```python
from build123d import *

# Parameters (mm, degrees)
F2_DEPTH = 12.7
F3_R     = 9.525
F4_DEPTH = 12.7
F5_W     = 60
F5_H     = 12.7
F5_W_2   = 12.7
F5_H_2   = 60
F6_DEPTH = 19.05
F7_W     = 203.2
F7_H     = 203.2
F7_W_2   = 184.15
F7_H_2   = 184.15
F8_DEPTH = 152.4


with BuildPart() as f2:
    # F1 (on offset) → F2 (new body)
    with BuildSketch(Plane.XY.offset(304.8)):
        Polygon((50.8, 17.960512), (68.760512, 0), (477.339488, 0), (495.3, 17.960512), (495.3, 337.639488), (477.339488, 355.6), (68.760512, 355.6), (50.8, 337.639488), align=None)
    extrude(amount=-F2_DEPTH)

    # F3 (on face) → F4 (cut)
    with BuildSketch(Plane.XY.offset(304.8)):
        with Locations((396.217286, 302.437495)):
            Circle(F3_R)
        with Locations((396.217286, 42.437495)):
            Circle(F3_R)
        with Locations((136.217286, 302.437495)):
            Circle(F3_R)
        with Locations((136.217286, 42.437495)):
            Circle(F3_R)
    extrude(amount=-F4_DEPTH, mode=Mode.SUBTRACT)

    # F5 (on face) → F6 (join)
    with BuildSketch(Plane.XY.offset(304.8)):
        with Locations((273.05, 331.7875)):
            Rectangle(F5_W, F5_H)
        with Locations((432.4, 172.4375)):
            Rectangle(F5_W_2, F5_H_2)
    extrude(amount=F6_DEPTH)

    # F7 (on face) → F8 (join)
    with BuildSketch(Plane(origin=(0, 0, 292.1), x_dir=(1, 0, 0), z_dir=(0, 0, -1))):
        with Locations((273.05, -177.8)):
            Rectangle(F7_W, F7_H)
        with Locations((273.05, -177.8)):
            Rectangle(F7_W_2, F7_H_2, mode=Mode.SUBTRACT)
    extrude(amount=F8_DEPTH)


solid = f2.part
```
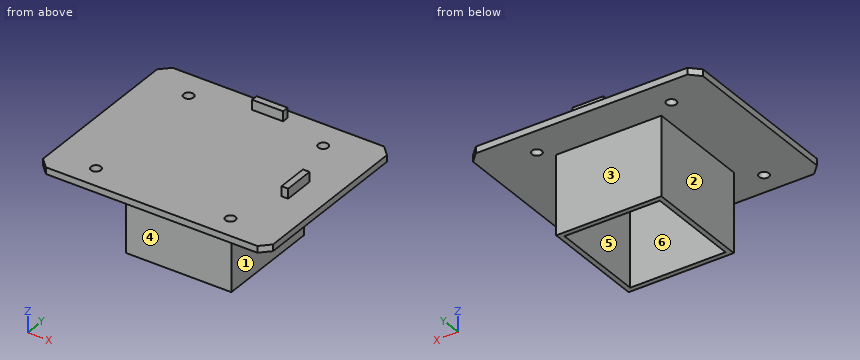
Design review of the part built by this model. Coordinates are the model's own, in mm. Face numbers are marked on the shaded views. A direction names the side the tool comes from. Round coordinates to 2 decimals unless told otherwise and drop trailing zeros. Write each loop counter-clockwise with the first axis right and the second up, starting at its lowest first coordinate (ties: lowest second). Pieces come first, ordered by that corner, then holes. Notation, with made-up numbers: (-27.75, 61) -> (0.25, 61) arc R15 cw to (0.25, 88) -> close; hole circle Ø8 at (84.5, 58.5). An arc over 180 degrees is marked (long way). Answer in a Markdown table with one row per item.
Q1. Take a section at C-C, the plane z = 177.5. State the section outline as (x, y) points (3 decimals).
The answers:
| item | result |
|---|---|
| outline | (171.45, 76.2) -> (374.65, 76.2) -> (374.65, 279.4) -> (171.45, 279.4) -> close; hole (180.975, 85.725) -> (365.125, 85.725) -> (365.125, 269.875) -> (180.975, 269.875) -> close |
Q2. Clearance check with flat-ended pins moving along their axes: pin 1 Ø10 at (y, z) = (79.5, 285.5) entering from -X; pin 2 Ø2 at (x, y) = (116, 230.5) entering from -Z; pin 3 Ø8 at (x, y) = (195.5, 119.5) entering from +Z. State where each tip first meets the part, or that it passes through.
The answers:
| item | result |
|---|---|
| pin 1 | x = 171.45 |
| pin 2 | z = 292.1 |
| pin 3 | z = 304.8 |
Q3. Take a section at D-D, the plane x = 197. State the section outline as (y, z) points (3 decimals).
The answers:
| item | result |
|---|---|
| outline | (0, 292.1) -> (76.2, 292.1) -> (76.2, 139.7) -> (85.725, 139.7) -> (85.725, 292.1) -> (269.875, 292.1) -> (269.875, 139.7) -> (279.4, 139.7) -> (279.4, 292.1) -> (355.6, 292.1) -> (355.6, 304.8) -> (0, 304.8) -> close |
Q4. To check wall thickness, follow L1, parallel to X at y = 256, z = 196 (3 decimals); L2, parallel to Y at x = 294, z = 182 (3 decimals); L3, parallel to Z at x = 394.5, y = 164. State the ranges of each line that lie inside material, in increasing order. Write a range as [from, to].
The answers:
| item | result |
|---|---|
| L1 | [171.45, 180.975], [365.125, 374.65] |
| L2 | [76.2, 85.725], [269.875, 279.4] |
| L3 | [292.1, 304.8] |
Q5. For the marked faces 1 and 2, list the 3-axis set-ups (+Z, -Z, +X, -X, +Y, -Y) from which the entire face can be reached by the end or side of a thin tool; tool diameter is ignored.
The answers:
| item | result |
|---|---|
| face 1 | -Z, +X, +Y, -Y |
| face 2 | -Z, -X, +Y, -Y |
Q6. Draft analysis for pull direction Y (two halves, no side actions). For the marked faces 3, 4, 5 and 6, state which applies: +Y half, -Y half, draft (parallel to the pull), parting line (faces both ways), or undercut.
The answers:
| item | result |
|---|---|
| face 3 | +Y half |
| face 4 | -Y half |
| face 5 | undercut |
| face 6 | undercut |
Q7. Take a section at A-A, the plane y = 233.5. State the section outline as (x, z) points (3 decimals).
The answers:
| item | result |
|---|---|
| outline | (50.8, 292.1) -> (171.45, 292.1) -> (171.45, 139.7) -> (180.975, 139.7) -> (180.975, 292.1) -> (365.125, 292.1) -> (365.125, 139.7) -> (374.65, 139.7) -> (374.65, 292.1) -> (495.3, 292.1) -> (495.3, 304.8) -> (50.8, 304.8) -> close |
